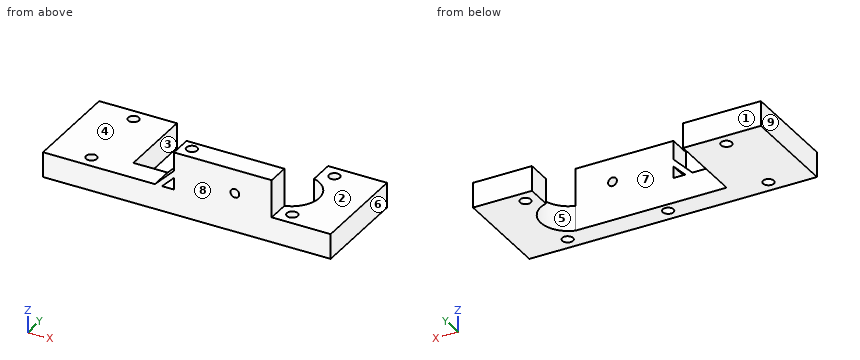
Autodesk Inventor part; units mm, degrees
ref_plane "YZ Plane" through (0, 0, 0) normal (1, 0, 0) x (0, 1, 0)
ref_plane "XZ Plane" through (0, 0, 0) normal (0, 1, 0) x (-1, 0, 0)
ref_plane "XY Plane" through (0, 0, 0) normal (0, 0, 1) x (1, 0, 0)
sketch "Esquisse1" plane through (0, 0, 0) normal (0, 0, 1) x (1, 0, 0)
  line L0 (30.1547, 20.0742) -> (30.1547, 11.0742)
  line L1 (30.1547, 11.0742) -> (49.0652, 11.0742)
  line L2 (49.0652, 11.0742) -> (49.0652, -11.0742)
  line L3 (49.0652, -11.0742) -> (-60.9348, -11.0742)
  line L4 (-60.9348, -11.0742) -> (-60.9348, -20.0742)
  line L5 (-60.9348, -20.0742) -> (53.6264, -20.0742)
  line L6 (53.6264, -20.0742) -> (53.6264, 20.0742)
  line L7 (53.6264, 20.0742) -> (30.1547, 20.0742)
  circle A0 centre (35.4871, 15.0742) radius 2.15
  circle A1 centre (-44.5129, -14.9258) radius 2.15
  circle A2 centre (-4.5129, -14.9258) radius 2.15
  circle A3 centre (35.4871, -14.9258) radius 2.15
  line L8 (30.1547, 11.0742) -> (30.1547, -11.0742)
  point P0 (0, 0)
extrude "Extrusion1" add sketch "Esquisse1" along normal blind 10
sketch "Esquisse2" plane through (0, 0, 10) normal (0, 0, 1) x (1, 0, 0)
  circle A0 centre (35.4871, -14.9258) radius 2.15
  circle A1 centre (-4.5129, -14.9258) radius 2.15
  circle A2 centre (-44.5129, -14.9258) radius 2.15
  circle A3 centre (35.4871, 15.0742) radius 2.15
  line L0 (30.1547, 20.0742) -> (30.1547, -11.0742)
  line L1 (30.1547, -11.0742) -> (-60.9348, -11.0742)
  line L2 (-60.9348, -11.0742) -> (-60.9348, -20.0742)
  line L3 (-60.9348, -20.0742) -> (53.6264, -20.0742)
  line L4 (53.6264, -20.0742) -> (53.6264, 20.0742)
  line L5 (53.6264, 20.0742) -> (30.1547, 20.0742)
  line L6 (-60.9348, -20.0742) -> (53.6264, -20.0742)
  line L7 (30.1547, -20.0742) -> (30.1547, -11.0742)
  line L8 (-60.9348, -20.0742) -> (53.6264, -20.0742)
  line L9 (-8.7922, -20.0742) -> (-8.7922, -11.0742)
  line L10 (30.1547, -11.0742) -> (-60.9348, -11.0742)
  point P0 (0, 0)
extrude "Extrusion2" add sketch "Esquisse2" along normal blind 15 contours L7 L3 L9 L1
sketch "Esquisse3" plane through (-60.9348, -11.0742, 0) normal (0, 1, 0) x (1, 0, 0)
  line L0 (91.0895, 0) -> (91.0895, -10)
  line L1 (91.0895, 0) -> (0, 0)
  line L2 (0, 0) -> (0, -10)
  line L3 (52.1426, -10) -> (0, -10)
  line L4 (52.1426, -10) -> (52.1426, -25)
  line L5 (91.0895, -25) -> (52.1426, -25)
  line L6 (91.0895, -10) -> (91.0895, -25)
  line L7 (91.0895, 0) -> (0, 0)
  line L8 (30.9674, 0) -> (30.9674, -10)
  point P0 (60.9348, 0)
extrude "Extrusion3" add sketch "Esquisse3" along normal blind 31 contours L8 L3 L2 L1
ref_plane "Plan de construction1" through (0, 0, 0) normal (0, 0, 1) x (1, 0, 0)
sketch "Esquisse4" plane through (0, 0, 0) normal (0, 0, 1) x (1, 0, 0)
  point P0 (0, 0)
sketch "Esquisse5" plane through (0, 0, 0) normal (0, 0, 1) x (1, 0, 0)
  circle A0 centre (-44.5129, 15.0742) radius 2.15
  point P0 (0, 0)
extrude "Extrusion4" cut sketch "Esquisse5" along normal blind 31
sketch "Esquisse6" plane through (-8.7922, -11.0742, 25) normal (0, 1, 0) x (1, 0, 0)
  line L0 (6.4293, 0) -> (2.1293, 0)
  line L1 (4.2793, 0) -> (4.2793, 25) construction
  line L2 (2.1293, 25) -> (6.4293, 25)
  line L3 (4.2793, 25) -> (4.2793, 9.5)
  line L4 (4.2793, 9.5) -> (24.2793, 9.5) construction
  circle A0 centre (24.2793, 9.5) radius 1.75
  point P0 (8.7922, 25)
  dimension "d8" = 15.5
  dimension "d9" = 20
  dimension "d10" = 3.5
extrude "Extrusion5" cut sketch "Esquisse6" against normal blind 10
sketch "Esquisse7" plane through (0, 0, 10) normal (0, 0, 1) x (1, 0, 0)
  line L0 (30.1547, -11.0742) -> (30.1547, -20.0742)
  line L1 (30.1547, 20.0742) -> (30.1547, -11.0742)
  arc A0 (30.1547, -11.0742) -> (30.1547, 10.0925) centre (27.156, -0.4909) ccw
  line L2 (30.1547, -11.0742) -> (-29.9674, -11.0742)
  line L3 (30.1547, -11.0742) -> (30.1547, 10.0925)
  point P0 (0, 0)
  dimension "d13" = 11
extrude "Extrusion6" cut sketch "Esquisse7" against normal blind 10
sketch "Esquisse8" plane through (-8.7922, -11.0742, 25) normal (0, 1, 0) x (1, 0, 0)
  line L0 (0, 15) -> (0, 0)
  line L1 (0, 7.5) -> (-7.5714, 15)
  line L2 (0, 15) -> (-21.1752, 15)
  line L3 (0, 10.3151) -> (-4.7295, 15)
  point P0 (8.7922, 25)
  dimension "d16" = 2
extrude "Extrusion7" add sketch "Esquisse8" against normal blind 9 contours L0 L1 L2 L3
properties part number "Aide_rotate"
Work out the finished part from the listing and answer in its coordinate system (mm). Face numbers are marked on the shaded views. A direction names the side the tool comes from. Give positions to 0.01 mm unless a question says otherwise; leave off trailing zeros. Write each loop counter-clockwise with the first axis right and the second up, starting at its lowest first coordinate (ties: lowest second). Pieces come first, ordered by that corner, then holes. Notation, with made-up numbers: (-32.75, 56.5) -> (22.25, 56.5) arc R14 ccw to (22.25, 68.5) -> close; hole circle Ø10 at (41.25, -25.75). An arc over 180 degrees is marked (long way). Write each question's results on one line, items separated by ' | '.
1. Find section A-A on y = -16. Determine the outline of the cut face in (x, z).
Data:
outline: (-60.93, 0) -> (-46.38, 0) -> (-46.38, 10) -> (-60.93, 10) -> close; (-42.65, 0) -> (-6.38, 0) -> (-6.38, 25) -> (-8.79, 25) -> (-8.79, 17.5) -> (-16.36, 10) -> (-42.65, 10) -> close; (-2.65, 0) -> (33.62, 0) -> (33.62, 10) -> (30.15, 10) -> (30.15, 25) -> (-2.65, 25) -> close; (37.35, 0) -> (53.63, 0) -> (53.63, 10) -> (37.35, 10) -> close; hole (-13.52, 10) -> (-8.79, 10) -> (-8.79, 14.68) -> close; hole circle Ø3.5 at (15.49, 15.5)
2. A tool of negligible diameter and unlimited length cuts with its end or side. For the marked faces 1, 2, 3, 4 and 5, from which of +Z, -Z, +X, -X, +Y, -Y can it reach the whole face along a straight path? Write none if from no direction.
Data:
face 1: +Z, -Z, -X, +Y | face 2: +Z, +X, +Y, -Y | face 3: +Z, -Z, +Y | face 4: +Z, -X, +Y, -Y | face 5: +Z, -Z
3. Find section B-B on y = -7. Determine the outline of the cut face in (x, z), and give its area (3 significant figures).
Data:
outline: (-60.93, 0) -> (-29.97, 0) -> (-29.97, 10) -> (-60.93, 10) -> close; (36.02, 0) -> (53.63, 0) -> (53.63, 10) -> (36.02, 10) -> close | area: 486 mm^2
4. Each of these flat-tipped pins is pushed along its axis until it touches: pin 1 Ø4.5 at (y, z) = (-15, 19) entering from +X; pin 2 Ø1.4 at (y, z) = (-16, 13.5) entering from -X; pin 3 Ø6 at (y, z) = (-17, 21.5) entering from -X; pin 4 Ø2 at (x, y) = (36, 6.5) entering from -Z. Where does it stop, or does it pass through?
Data:
pin 1: x = 30.15 | pin 2: x = -13.54 | pin 3: x = -8.79 | pin 4: z = 0
5. Straight lines are drawn through the part: L1, parallel to X at y = -15.5, z = 15.5; L2, parallel to Y at x = 22.5, z = 22.25; L3, parallel to Z at x = -49, y = -8.5. For each, find the intervals that lie inside material, in ascending order.
Data:
L1: -10.81 to -6.58, -2.44 to 13.74, 17.24 to 30.15 | L2: -20.07 to -11.07 | L3: 0 to 10
6. Determine the mould class of the marked faces 6, 7, 8 and 9 for opening direction X: +X half, -X half, draft (parallel to the pull), parting line (faces both ways), or undercut.
Data:
face 6: +X half | face 7: undercut | face 8: draft | face 9: -X half
7. Find section C-C on z = 5.25. Determine the outline of the cut face in (x, y).
Data:
outline: (-60.93, -20.07) -> (53.63, -20.07) -> (53.63, 20.07) -> (30.15, 20.07) -> (30.15, 10.09) arc R11 cw to (30.15, -11.07) -> (-29.97, -11.07) -> (-29.97, 19.93) -> (-60.93, 19.93) -> close; hole circle Ø4.3 at (-44.51, -14.93); hole circle Ø4.3 at (-44.51, 15.07); hole circle Ø4.3 at (-4.51, -14.93); hole circle Ø4.3 at (35.49, -14.93); hole circle Ø4.3 at (35.49, 15.07)
8. Find section D-D on x = -3.5. Determine the outline of the cut face in (y, z), and give its area (3 significant figures).
Data:
outline: (-20.07, 0) -> (-16.82, 0) -> (-16.82, 25) -> (-20.07, 25) -> close; (-13.03, 0) -> (-11.07, 0) -> (-11.07, 25) -> (-13.03, 25) -> close | area: 130 mm^2
